```python
from build123d import *

# Parameters (mm, degrees)
SKETCH1_W           = 304.8
SKETCH1_H           = 152.4
BOSS_EXTRUDE1_DEPTH = 0.79375


with BuildPart() as part:
    # Sketch1 → Boss-Extrude1 (new body, symmetric)
    with BuildSketch(Plane.XY):
        Rectangle(SKETCH1_W, SKETCH1_H)
        Polygon((-127, 50.8), (-127, -50.8), (-25.4, 0), align=None, mode=Mode.SUBTRACT)
        Polygon((-70.203873372, 50.8), (70.203873372, 50.8), (0, 15.698063314), align=None, mode=Mode.SUBTRACT)
        Polygon((0, -15.698063314), (-70.203873372, -50.8), (70.203873372, -50.8), align=None, mode=Mode.SUBTRACT)
        Polygon((25.4, 0), (127, 50.8), (127, -50.8), align=None, mode=Mode.SUBTRACT)
    extrude(amount=BOSS_EXTRUDE1_DEPTH, both=True)


solid = part.part
```
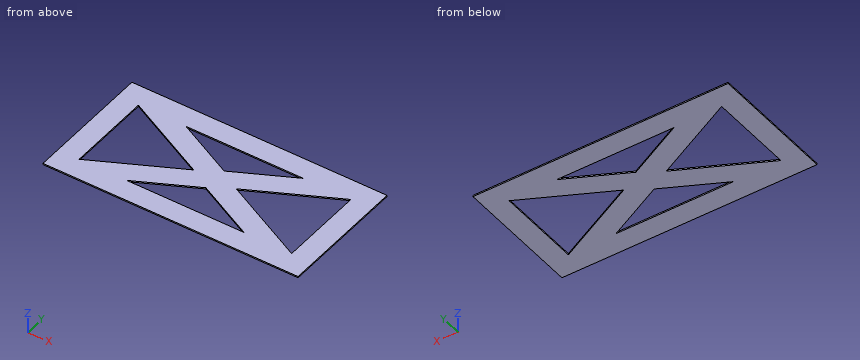
Work out the finished part from the listing and answer in its coordinate system (mm). Round coordinates to 2 decimals unless told otherwise and drop trailing zeros. Order: outer loops, then holes, each group sorted by start corner. A loop starts at its lowest first (then second) coordinate and runs counter-clockwise, first axis right, second up.
Q1. A cutting plane is placed at A-A, the plane x = -91. Determine the outline of the cut face in (y, z), then the cut area to 3 significant figures.
Solution:
outline: (-76.2, -0.79) - (-32.8, -0.79) - (-32.8, 0.79) - (-76.2, 0.79) - close; (32.8, -0.79) - (76.2, -0.79) - (76.2, 0.79) - (32.8, 0.79) - close
area: 138 mm2
Q2. Find the intervals of material crossed by line 1 along X through (y, z) = (0, 0.4); line 2 along Y through (x, z) = (31, -0.4); line 3 along X through (y, z) = (-7.5, 0.7), in increasing order.
Solution:
line 1: x = -152.4 to -127, -25.4 to 25.4, 127 to 152.4
line 2: y = -76.2 to -50.8, -31.2 to -2.8, 2.8 to 31.2, 50.8 to 76.2
line 3: x = -152.4 to -127, -40.4 to 40.4, 127 to 152.4
Q3. A cutting plane is placed at B-B, the plane z = -0.15. Determine the outline of the cut face in (x, y).
Solution:
outline: (-152.4, -76.2) - (152.4, -76.2) - (152.4, 76.2) - (-152.4, 76.2) - close; hole (-127, -50.8) - (-25.4, 0) - (-127, 50.8) - close; hole (-70.2, -50.8) - (70.2, -50.8) - (0, -15.7) - close; hole (-70.2, 50.8) - (0, 15.7) - (70.2, 50.8) - close; hole (25.4, 0) - (127, -50.8) - (127, 50.8) - close
Q4. A cutting plane is placed at D-D, the plane y = 25. Determine the outline of the cut face in (x, z), then the cut area to 3 significant figures.
Solution:
outline: (-152.4, -0.79) - (-127, -0.79) - (-127, 0.79) - (-152.4, 0.79) - close; (-75.4, -0.79) - (-18.6, -0.79) - (-18.6, 0.79) - (-75.4, 0.79) - close; (18.6, -0.79) - (75.4, -0.79) - (75.4, 0.79) - (18.6, 0.79) - close; (127, -0.79) - (152.4, -0.79) - (152.4, 0.79) - (127, 0.79) - close
area: 261 mm2
Q5. A cutting plane is placed at C-C, the plane x = -41. Determine the outline of the cut face in (y, z).
Solution:
outline: (-76.2, -0.79) - (-50.8, -0.79) - (-50.8, 0.79) - (-76.2, 0.79) - close; (-36.2, -0.79) - (-7.8, -0.79) - (-7.8, 0.79) - (-36.2, 0.79) - close; (7.8, -0.79) - (36.2, -0.79) - (36.2, 0.79) - (7.8, 0.79) - close; (50.8, -0.79) - (76.2, -0.79) - (76.2, 0.79) - (50.8, 0.79) - close
